Geometry: final body of the model. Coordinates: model frame, mm. Face numbers are marked on the shaded views. A direction names the side the tool comes from. Coordinates: 2 decimals unless noted, no trailing zeros. Write each loop counter-clockwise with the first axis right and the second up, starting at its lowest first coordinate (ties: lowest second). Pieces come first, ordered by that corner, then holes. Notation, with made-up numbers: (-39.5, 67) -> (13.5, 67) arc R11 cw to (13.5, 78) -> close; hole circle Ø1 at (-14, 46). An arc over 180 degrees is marked (long way). Answer as a JSON object with one key per item and string values. Group by question number.
```python
from build123d import *

# Parameters (mm, degrees)
F1_DEPTH = 63.5
F0_W     = 25.1418616311
F0_H     = 15.24
F2_DEPTH = 25.4
F3_DEPTH = 7.62
F5_R     = 5.08
F6_R     = 5.08
F7_R     = 5.08
F8_R     = 5.08


with BuildPart() as f1:
    # F0 (on Front) → F1 (new body, symmetric)
    with BuildSketch(Plane.XZ):
        Polygon((-41.275, -9.525), (41.275, -9.525), (41.275, 9.525), (26.035, 9.525), (-41.275, 9.525), align=None)
    extrude(amount=F1_DEPTH, both=True)

    # F0 (on Front) → F2 (join, symmetric)
    with BuildSketch(Plane.XZ):
        with BuildLine():
            Line((26.035, 9.525), (41.275, 9.525))
            Line((41.275, 9.525), (41.275, 36.195))
            ThreePointArc((41.275, 36.195), (44.2507951031, 43.3792048969), (51.435, 46.355))
            Line((51.435, 46.355), (60.325, 46.355))
            Line((60.325, 46.355), (60.325, 61.595))
            Line((60.325, 61.595), (51.435, 61.595))
            ThreePointArc((51.435, 61.595), (33.4744877579, 54.1555122421), (26.035, 36.195))
            Line((26.035, 36.195), (26.035, 9.525))
        make_face()
        with Locations((72.8959308155, 53.975)):
            Rectangle(F0_W, F0_H)
    extrude(amount=F2_DEPTH, both=True)

    # F0 (on Front) → F3 (join, symmetric)
    with BuildSketch(Plane.XZ):
        with BuildLine():
            add(Edge.make_bspline(
                [(-41.275, 9.525), (-24.5270843474, 44.4972960267), (2.2869093497, 62.1685317942), (51.435, 61.595)],
                knots=[0, 0, 0, 0, 106.3316932998, 106.3316932998, 106.3316932998, 106.3316932998], degree=3))
            Line((-41.275, 9.525), (26.035, 9.525))
            Line((26.035, 9.525), (26.035, 36.195))
            ThreePointArc((26.035, 36.195), (33.4744877579, 54.1555122421), (51.435, 61.595))
        make_face()
    extrude(amount=F3_DEPTH, both=True)

    # F0 (on Front) → F4 (revolve)
    with BuildSketch(Plane.XZ):
        Polygon((85.4668616311, 68.6612712564), (85.4668616311, 61.595), (85.4668616311, 46.355), (85.4668616311, 40.2132712564), (111.125, 40.2132712564), (111.125, 68.6612712564), align=None)
    revolve(axis=Axis((85.4668616311, 0, 57.5081356282), (0, 0, 1)))

    # F5
    f5_edges = [f1.edges().sort_by_distance(p)[0] for p in [
        (41.275, -63.5, 0),
    ]]
    fillet(f5_edges, radius=F5_R)

    # F6
    f6_edges = [f1.edges().sort_by_distance(p)[0] for p in [
        (-41.275, -63.5, 0),
    ]]
    fillet(f6_edges, radius=F6_R)

    # F7
    f7_edges = [f1.edges().sort_by_distance(p)[0] for p in [
        (41.275, 63.5, 0),
    ]]
    fillet(f7_edges, radius=F7_R)

    # F8
    f8_edges = [f1.edges().sort_by_distance(p)[0] for p in [
        (-41.275, 63.5, 0),
    ]]
    fillet(f8_edges, radius=F8_R)


solid = f1.part
```
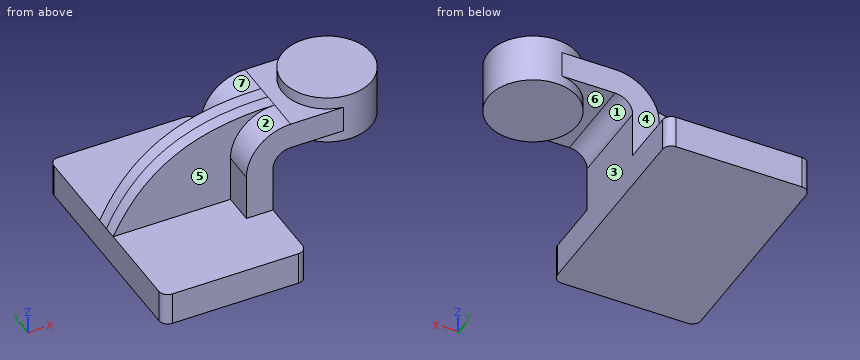
Item 1: Ray query, L1, parallel to Z at x = 13.5, y = -17.5 (3 decimals); L2, parallel to Y at x = 8, z = 29; L3, parallel to Z at x = 74.5, y = 1. Return the intervals inside material, ascending. Write a range as [from, to].
Item 2: Mould query, pull axis X, two halves, no side actions, for the marked faces 5, 6 and 7. Classes: +X half, -X half, draft (parallel to the pull), parting line (faces both ways), or undercut.
Item 3: Section A-A on y = 23. Output: boundary loops of the cut face in (x, z) (3 decimals), then the cut area to 3 significant figures.
Item 4: Set-up query: the marked faces 1, 2, 3 and 4. Return all of +Z, -Z, +X, -X, +Y, -Y with unobstructed straight access to the full face (end or side cutting, diameter ignored); none if empty.
Item 5: Contact query for flat-ended pins moving along their axis: pin 1 (1.5 mm diameter, centred on x = -3, z = 16.5, fed in from +Y); pin 2 (8 mm diameter, centred on y = -25.5, z = 2.5, fed in from +X) (3 decimals); pin 3 (14 mm diameter, centred on y = -18.5, z = 25, fed in from -X) (3 decimals). Output: stop coordinate, or through.
Answer sheet:
{
 "1": {"L1": "z = [-9.525, 9.525]", "L2": "y = [-7.62, 7.62]", "L3": "z = [40.21, 68.66]"},
 "2": {"face 5": "draft", "face 6": "undercut", "face 7": "-X half"},
 "3": {"outline": "(-41.275, -9.525) -> (41.275, -9.525) -> (41.275, 36.195) arc R10.16 cw to (51.435, 46.355) -> (74.094, 46.355) -> (74.094, 40.213) -> (96.84, 40.213) -> (96.84, 68.661) -> (74.094, 68.661) -> (74.094, 61.595) -> (51.435, 61.595) arc R25.4 ccw to (26.035, 36.195) -> (26.035, 9.525) -> (-41.275, 9.525) -> close", "area": "3,400 mm^2"},
 "4": {"face 1": "-Z, +Y, -Y", "face 2": "+Z, -X, -Y", "face 3": "-Z, +X, +Y, -Y", "face 4": "+Z, -X, +Y"},
 "5": {"pin 1": "stops at y = 7.62", "pin 2": "stops at x = 41.275", "pin 3": "stops at x = 26.035"}
}
